Model file for the job. Use its own axes, mm. A direction names the side the tool comes from. Coordinates: 2 decimals unless noted, no trailing zeros. Order: outer loops, then holes, each group sorted by start corner. A loop starts at its lowest first (then second) coordinate and runs counter-clockwise, first axis right, second up. Notation, with made-up numbers: (56, -36.5) - (70, -36.5) arc R22 cw to (70, -5.5) - close; hole circle Ø11 at (-34.5, 37). An arc over 180 degrees is marked (long way). Put each result on its own line as item: value. Start each with the question number.
```python
from build123d import *

# Parameters (mm, degrees)
F1_DEPTH  = 25.4
F3_DEPTH  = 25.4
F3_FACE_W = 25.4
F3_FACE_H = 18.81851
F4_DEPTH  = 0.268369


with BuildPart() as f1:
    # F0 (on Front) → F1 (new body)
    with BuildSketch(Plane.XZ):
        Polygon((0, 31.558946), (-38.099521, 31.75), (-38.099521, 0), (0, 0), align=None)
    extrude(amount=F1_DEPTH)

    # F2 (on Right) → F3 (cut)
    with BuildSketch(Plane.YZ):
        Polygon((-25.44473, 6.083318), (-6.581489, 31.482631), (-25.631489, 31.482631), align=None)
    extrude(amount=-F3_DEPTH, mode=Mode.SUBTRACT)

    # F3_face (on face) → F4 (cut, through all)
    with BuildSketch(Plane(origin=(-12.7, -15.990745, 31.482631), x_dir=(1, 0, 0), z_dir=(0, 0, -1))):
        Rectangle(F3_FACE_W, F3_FACE_H)
    extrude(amount=-F4_DEPTH, mode=Mode.SUBTRACT)


solid = f1.part
```
Item 1: Slice it at C-C, the plane z = 17. Give the cut face in (x, y).
Item 2: Wall check: line 1 along Z through (x, y) = (-1.5, -3.75); line 2 along X through (y, z) = (-21.75, 20); line 3 along Y through (x, z) = (-18, 23.5). Give the ranges that are in metal, low to high.
Item 3: Slice it at B-B, the plane y = -21.5. Give the cut face in (x, z).
Item 4: Flat gauge pin, fed straight in: pin 1 Ø10 at (x, y) = (-21.5, -15.5) entering from +Z. Where does the tip first touch, or does it go through?
Item 5: 3-axis set-ups, long thin cutter, end or side, ignore diameter. For faces 1 (the face through (-25.4, -20, 24)), 2 (the face through (-19, -13, 0)): which of +Z, -Z, +X, -X, +Y, -Y reach the whole face in a straight line?
Here are the results:
1. outline: (-38.1, -25.4) - (-25.4, -25.4) - (-25.4, -17.34) - (0, -17.34) - (0, 0) - (-38.1, 0) - close
2. line 1: z = 0 to 31.57
2. line 2: x = -38.1 to -25.4
2. line 3: y = -12.51 to 0
3. outline: (-38.1, 0) - (0, 0) - (0, 11.39) - (-25.4, 11.39) - (-25.4, 31.69) - (-38.1, 31.75) - close
4. pin 1: stops at z = 31.69
5. face 1: +Z, +X, -Y
5. face 2: -Z, +X, -X, +Y, -Y
